For this review, take the finished solid that the model builds, in its own axes (mm). A direction names the side the tool comes from. Give positions to 0.01 mm unless a question says otherwise; leave off trailing zeros. Order: outer loops, then holes, each group sorted by start corner. A loop starts at its lowest first (then second) coordinate and runs counter-clockwise, first axis right, second up. Notation, with made-up numbers: (34.25, -8) -> (91.25, -8) arc R33 ccw to (91.25, 31) -> close; hole circle Ø4 at (74.25, -0.5). An arc over 180 degrees is marked (long way). Use CSV: the item, a comma, the result in double quotes. Start each with the question number.
```python
from build123d import *

# Parameters (mm, degrees)
SKETCH3_W                                           = 116.586
SKETCH3_H                                           = 72.644
BOSS_EXTRUDE1_DEPTH                                 = 5.969
BOSS_EXTRUDE2_DEPTH                                 = 36.322
BOSS_EXTRUDE3_DEPTH                                 = 9.652
CUT_EXTRUDE1_REACH                                  = 108.219
SKETCH6_R                                           = 11.938
CBORE_FOR_00_BINDING_HEAD_MACHINE_SCREW_D           = 7.366
CBORE_FOR_00_BINDING_HEAD_MACHINE_SCREW_CBORE_D     = 14.224
CBORE_FOR_00_BINDING_HEAD_MACHINE_SCREW_CBORE_DEPTH = 4.826
SKETCH9_R                                           = 16.637
CUT_EXTRUDE2_DEPTH                                  = 93.852634798


with BuildPart() as part:
    # Sketch3 → Boss-Extrude1 (new, symmetric)
    with BuildSketch(Plane(origin=(0, 0, 0), x_dir=(1, 0, 0), z_dir=(0, 1, 0))):
        Rectangle(SKETCH3_W, SKETCH3_H)
    extrude(amount=BOSS_EXTRUDE1_DEPTH, both=True)

    # Sketch4 → Boss-Extrude2 (add, symmetric)
    with BuildSketch(Plane.XY):
        Polygon((-31.135464213, 5.969), (-20.193, 75.057), (20.193, 75.057), (31.135464213, 5.969), align=None)
        Polygon((-23.403173679, 12.573), (-14.552651153, 68.453), (14.552651153, 68.453), (23.403173679, 12.573), align=None, mode=Mode.SUBTRACT)
    extrude(amount=BOSS_EXTRUDE2_DEPTH, both=True)

    # Sketch5 → Boss-Extrude3 (add)
    with BuildSketch(Plane(origin=(0, 0, -3.302), x_dir=(-1, 0, 0), z_dir=(0, 0, -1))):
        Polygon((-20.193, 75.057), (-58.293, 5.969), (-31.135464213, 5.969), align=None)
    boss_extrude3 = extrude(amount=-BOSS_EXTRUDE3_DEPTH)

    # Mirror1: Boss-Extrude3 across plane
    add(boss_extrude3.mirror(Plane(origin=(0, 0, 0), x_dir=(0, 0, 1), z_dir=(1, 0, 0))))

    # Sketch6 → Cut-Extrude1 (cut, up to next)
    with BuildSketch(Plane(origin=(0, 75.057, 0), x_dir=(1, 0, 0), z_dir=(0, 1, 0)), mode=Mode.PRIVATE) as cut_extrude1_sk1:
        with Locations(Location((-0.127, 0, 0), (0, 0, 270))):
            Circle(SKETCH6_R)
    cut_extrude1_tool1 = extrude(cut_extrude1_sk1.sketch, amount=-CUT_EXTRUDE1_REACH, mode=Mode.PRIVATE) & part.part
    add(cut_extrude1_tool1.solids().sort_by_distance((-0.127, 75.057, 0))[0], mode=Mode.SUBTRACT)

    # CBORE for #00 Binding Head Machine Screw1 (through all)
    with Locations(Plane(origin=(-44.069, 5.969, 22.5984117), x_dir=(0, 0, 1), z_dir=(0, 1, 0))):
        with Locations((0, 0), (0, 88.138), (-45.212, 88.138), (-45.212, 0)):
            CounterBoreHole(CBORE_FOR_00_BINDING_HEAD_MACHINE_SCREW_D / 2, CBORE_FOR_00_BINDING_HEAD_MACHINE_SCREW_CBORE_D / 2, CBORE_FOR_00_BINDING_HEAD_MACHINE_SCREW_CBORE_DEPTH)

    # Sketch9 → Cut-Extrude2 (cut, through all)
    with BuildSketch(Plane(origin=(0, 12.573, 0), x_dir=(1, 0, 0), z_dir=(0, 1, 0))):
        with Locations(Location((0, 0, 0), (0, 0, 270))):
            Circle(SKETCH9_R)
    extrude(amount=-CUT_EXTRUDE2_DEPTH, mode=Mode.SUBTRACT)


solid = part.part
```
1. For faces 5 (the face through (18.916, 40.904, 0.509)), 6 (the face through (41, 1.143, -20)), 7 (the face through (-37, 28, 6.35)), 8 (the face through (37, 28, -3.302)), list the 3-axis set-ups (+Z, -Z, +X, -X, +Y, -Y) from which the entire face can be reached by the end or side of a thin tool; tool diameter is ignored.
2. Clearance check with flat-ended pins moving along their axes: P1, Ø12, axis at y = 34.5, z = 16, coming from the +X side; P2, Ø11.5, axis at x = 44.07, z = 22.6, coming from the +Y side; P3, Ø1, axis at y = 23, z = -20, coming from the +X side. State where each tip first meets the part, or that it passes through.
3. Draft analysis for pull direction X (two halves, no side actions). For faces 1 (the face through (25.588, 40.997, -19.581)), 2 (the face through (-25.74, 40.03, -19.58)), 3 (the face through (46.21, 3.59, -15.83)), 4 (the face through (37, 28, 6.35)), state which applies: +X half, -X half, draft (parallel to the pull), parting line (faces both ways), or undercut.
4. Consider section D-D (y = 45). State the section outline as (x, z) points, plus the area to 3 significant figures.
5. To check wall thickness, follow L1, parallel to X at y = 0.75, z = 0; L2, parallel to Y at x = 1, z = -23; L3, parallel to Y at x = 51, z = 12. State the ranges of each line that lie inside material, in increasing order. Write a range as [from, to].
6. Consider section A-A (z = 0). State the section outline as (x, y) points (3 decimals), plus the area to 3 significant figures.
7. Consider section C-C (x = 5). State the section outline as (y, z) points, plus the area to 3 significant figures.
8. Consider section B-B (y = 24.5). State the section outline as (x, z) points.
Answer list:
1,face 5,"+Z, -Z"
1,face 6,"+Y"
1,face 7,"+Z, -X, +Y"
1,face 8,"-Z, +X, +Y"
2,P1,"x = 27.57"
2,P2,"y = 1.14"
2,P3,"x = 28.52"
3,face 1,"+X half"
3,face 2,"-X half"
3,face 3,"undercut"
3,face 4,"draft"
4,outline,"(-36.77, -3.3) -> (-24.95, -3.3) -> (-24.95, -36.32) -> (-18.27, -36.32) -> (-18.27, 36.32) -> (-24.95, 36.32) -> (-24.95, 6.35) -> (-36.77, 6.35) -> close; (18.27, -36.32) -> (24.95, -36.32) -> (24.95, -3.3) -> (36.77, -3.3) -> (36.77, 6.35) -> (24.95, 6.35) -> (24.95, 36.32) -> (18.27, 36.32) -> close"
4,area,"1,200 mm2"
5,L1,"[-58.29, -16.64], [16.64, 58.29]"
5,L2,"[-5.97, 12.57], [68.45, 75.06]"
5,L3,"[-5.97, 5.97]"
6,outline,"(-58.293, -5.969) -> (-16.637, -5.969) -> (-16.637, 12.573) -> (-23.403, 12.573) -> (-14.553, 68.453) -> (-12.065, 68.453) -> (-12.065, 75.057) -> (-20.193, 75.057) -> (-58.293, 5.969) -> close; (11.811, 68.453) -> (14.553, 68.453) -> (23.403, 12.573) -> (16.637, 12.573) -> (16.637, -5.969) -> (58.293, -5.969) -> (58.293, 5.969) -> (20.193, 75.057) -> (11.811, 75.057) -> close"
6,area,"3,920 mm2"
7,outline,"(-5.97, -36.32) -> (12.57, -36.32) -> (12.57, -15.87) -> (-5.97, -15.87) -> close; (-5.97, 15.87) -> (12.57, 15.87) -> (12.57, 36.32) -> (-5.97, 36.32) -> close; (68.45, -36.32) -> (75.06, -36.32) -> (75.06, -10.78) -> (68.45, -10.78) -> close; (68.45, 10.78) -> (75.06, 10.78) -> (75.06, 36.32) -> (68.45, 36.32) -> close"
7,area,"1,100 mm2"
8,outline,"(-48.07, -3.3) -> (-28.2, -3.3) -> (-28.2, -36.32) -> (-21.51, -36.32) -> (-21.51, 36.32) -> (-28.2, 36.32) -> (-28.2, 6.35) -> (-48.07, 6.35) -> close; (21.51, -36.32) -> (28.2, -36.32) -> (28.2, -3.3) -> (48.07, -3.3) -> (48.07, 6.35) -> (28.2, 6.35) -> (28.2, 36.32) -> (21.51, 36.32) -> close"
